For this review, take the finished solid that the model builds, in its own axes (mm). A direction names the side the tool comes from. Round coordinates to 2 decimals unless told otherwise and drop trailing zeros. Order: outer loops, then holes, each group sorted by start corner. A loop starts at its lowest first (then second) coordinate and runs counter-clockwise, first axis right, second up. Notation, with made-up numbers: M 38.25,-32.5 L 57.25,-32.5 A21 ccw 57.25,-3.5 Z; hole C 24,10 d5. An arc over 180 degrees is marked long. Put each result on its own line as item: value.
Autodesk Inventor part; units mm, degrees
ref_plane "YZ Plane" through (0, 0, 0) normal (1, 0, 0) x (0, 1, 0)
ref_plane "XZ Plane" through (0, 0, 0) normal (0, 1, 0) x (-1, 0, 0)
ref_plane "XY Plane" through (0, 0, 0) normal (0, 0, 1) x (1, 0, 0)
sketch "草图2" plane through (0, 0, 0) normal (0, 1, 0) x (-1, 0, 0)
  line L0 (29.7873, 9.5105) -> (-28.2127, 9.5105)
  line L1 (-28.2127, 9.5105) -> (-48.2127, 0.5105)
  line L2 (-48.2127, 0.5105) -> (-48.2127, -8.4895)
  line L3 (-48.2127, -8.4895) -> (29.7873, -8.4895)
  line L4 (29.7873, -8.4895) -> (29.7873, 9.5105)
  dimension "d3" = 9
  dimension "d4" = 78
  dimension "d5" = 18
  dimension "d6" = 58
extrude "拉伸1" add sketch "草图2" along normal mid plane 48
sketch "草图3" plane through (48.2127, 24, -8.4895) normal (0, 0, -1) x (-1, 0, 0)
  line L0 (78, -48) -> (78, 0)
  line L1 (0, 0) -> (78, 0)
  line L2 (0, -48) -> (0, 0)
  line L3 (78, -48) -> (0, -48)
  line L4 (0, -48) -> (0, 0)
  line L5 (0, -33) -> (12, -33)
  line L6 (12, -33) -> (12, -15)
  line L7 (12, -15) -> (0, -15)
  line L8 (0, -15) -> (0, -33)
  point P0 (48.2127, -24)
  point P1 (0, -24)
  point P2 (0, -24)
  point P3 (0, -24)
  dimension "d9" = 18
  dimension "d10" = 12
extrude "拉伸2" cut sketch "草图3" against normal up to surface contours L2 L7 L6 L5 surface through (28.2127, 0, 9.5105) normal (0.4103647, 0, 0.9119215)
sketch "草图4" plane through (0, 24, 0) normal (0, 1, 0) x (1, 0, 0)
  line L0 (28.2127, -9.5105) -> (48.2127, -0.5105)
  line L1 (48.2127, -0.5105) -> (48.2127, 8.4895)
  line L2 (48.2127, 8.4895) -> (-29.7873, 8.4895)
  line L3 (-29.7873, 8.4895) -> (-29.7873, -9.5105)
  line L4 (-29.7873, -9.5105) -> (28.2127, -9.5105)
  line L5 (28.2127, -9.5105) -> (-29.7873, -9.5105)
  line L6 (-29.7873, -9.5105) -> (-29.7873, -30.5105)
  arc A0 (-29.7873, -30.5105) -> (6.2127, -30.5105) centre (-11.7873, -30.5105) ccw
  line L7 (6.2127, -30.5105) -> (6.2127, -9.5105)
  circle A1 centre (-11.7873, -30.5105) radius 9
  point P0 (0, 0)
  dimension "d13" = 39
  dimension "d14" = 18
  dimension "d15" = 18
extrude "拉伸3" add sketch "草图4" against normal blind 12 contours L7 A0 L6 L4
mirror "镜像1" about plane through (0, 0, 0) normal (0, 1, 0) of "拉伸3"
sketch "草图5" plane through (28.2127, -24, 9.5105) normal (0, 0, 1) x (1, 0, 0)
  line L0 (-58, 12) -> (-22, 12)
  line L1 (-22, 12) -> (-22, 0)
  line L2 (0, 0) -> (-22, 0)
  line L3 (0, 48) -> (0, 0)
  line L4 (-22, 48) -> (0, 48)
  line L5 (-22, 48) -> (-22, 36)
  line L6 (-22, 36) -> (-58, 36)
  line L7 (-58, 12) -> (-58, 36)
  line L8 (-16, 18) -> (-43, 18)
  arc A0 (-43, 30) -> (-43, 18) centre (-43, 24) ccw
  line L9 (-43, 30) -> (-16, 30)
  arc A1 (-16, 18) -> (-16, 30) centre (-16, 24) ccw
  point P0 (-28.2127, 24)
  point P1 (-58, 24)
  dimension "d18" = 6
  dimension "d19" = 27
  dimension "d20" = 15
extrude "拉伸4" cut sketch "草图5" against normal up to surface (18 mm away) contours L8 A0 L9 A1
(1) Add section C-C on z = -4. Give the boundary of the cut face in (x, y), then the cut area to 3 significant figures.
A:
outline: M -29.79,-24 L 48.21,-24 L 48.21,-9 L 36.21,-9 L 36.21,9 L 48.21,9 L 48.21,24 L -29.79,24 Z; hole M -14.79,-6 L 12.21,-6 A6 ccw 12.21,6 L -14.79,6 A6 ccw Z
area: 3,090 mm2
(2) Add section B-B on y = 0. Give the boundary of the cut face in (x, z).
A:
outline: M -29.79,-8.49 L -20.79,-8.49 L -20.79,9.51 L -29.79,9.51 Z; M 18.21,-8.49 L 36.21,-8.49 L 36.21,5.91 L 28.21,9.51 L 18.21,9.51 Z
(3) To check wall thickness, follow L1, parallel to Y at x = -10.5, z = 1; L2, parallel to Y at x = -2, z = 13; L3, parallel to Z at x = 12, y = -17. State the ranges of each line that lie inside material, in increasing order.
A:
L1: y = -24 to -6, 6 to 24
L2: y = -24 to -12, 12 to 24
L3: z = -8.49 to 9.51
(4) Add section D-D on y = -19. Give the boundary of the cut face in (x, z), then the cut area to 3 significant figures.
A:
outline: M -29.79,-8.49 L 48.21,-8.49 L 48.21,0.51 L 28.21,9.51 L 6.21,9.51 L 6.21,30.51 A18 ccw -29.79,30.51 Z; hole C -11.79,30.51 d18
area: 2,320 mm2
(5) For faces 4 (the face through (42, 9, -3)), 5 (the face through (-12, 12, 20)), 6 (the face through (6.213, 18, 20)), list the 3-axis set-ups (+Z, -Z, +X, -X, +Y, -Y) from which the entire face can be reached by the end or side of a thin tool; tool diameter is ignored.
A:
face 4: +Z, -Z, +X
face 5: +Z, +X, -X
face 6: +Z, +X, +Y, -Y
(6) Insertion check: pin 1 Ø13 at (y, z) = (-16.5, 21.5) entering from +X; pin 2 Ø10 at (x, y) = (-2.5, -12) entering from +Z; pin 3 Ø11.5 at (y, z) = (-0.5, -2) entering from +X. Each pin has a flat end and moves straight along its axis. Give the tip position at first contact, or say it passes through.
A:
pin 1: stops at x = 6.21
pin 2: stops at z = 47.99
pin 3: stops at x = 36.21
(7) Draft analysis for pull direction Y (two halves, no side actions). For faces 1 (the face through (-7.634, 18.084, 38.495)), 2 (the face through (1, -24, 13)), 3 (the face through (5, 10, 9.51)), state which applies: released by +Y, released by -Y, zero draft, split by the parting line, or undercut.
A:
face 1: zero draft
face 2: released by -Y
face 3: undercut
(8) Add section A-A on x = 8.5. Give the boundary of the cut face in (y, z).
A:
outline: M -24,-8.49 L -6,-8.49 L -6,9.51 L -24,9.51 Z; M 6,-8.49 L 24,-8.49 L 24,9.51 L 6,9.51 Z
